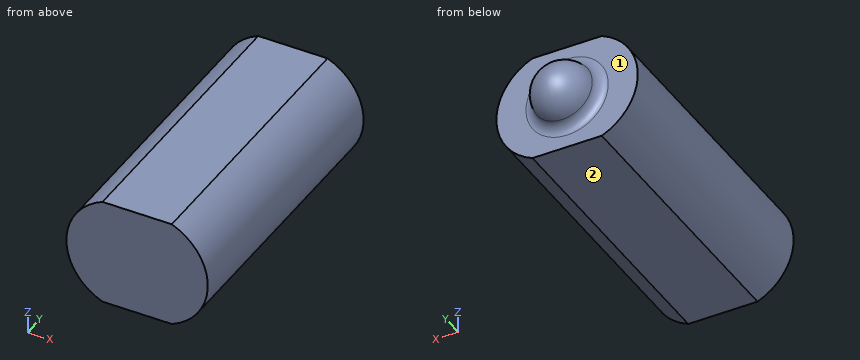
```python
from build123d import *

# Parameters (mm, degrees)
BOSS_EXTRUDE1_DEPTH = 80


with BuildPart() as part:
    # Sketch1 → Boss-Extrude1 (new body)
    with BuildSketch(Plane(origin=(0, 0, 0), x_dir=(1, 0, 0), z_dir=(0, 1, 0))):
        with BuildLine():
            Line((-9.791248996, 15.25), (9.791248996, 15.25))
            ThreePointArc((9.791248996, 15.25), (20, 0), (9.791248996, -15.25))
            Line((9.791248996, -15.25), (-9.791248996, -15.25))
            ThreePointArc((-9.791248996, -15.25), (-20, 0), (-9.791248996, 15.25))
        make_face()
    extrude(amount=BOSS_EXTRUDE1_DEPTH)

    # Sketch4 → Revolve1 (revolve)
    with BuildSketch(Plane(origin=(0, 0, 0), x_dir=(0, 0, -1), z_dir=(1, 0, 0))):
        with BuildLine():
            Line((0, 80), (11.641855063, 80))
            ThreePointArc((11.641855063, 80), (9.61766545, 80.745389743), (8.560304848, 82.625532826))
            ThreePointArc((8.560304848, 82.625532826), (5.623040011, 87.848422876), (0, 89.919057131))
            Line((0, 89.919057131), (0, 80))
        make_face()
    revolve(axis=Axis((0, 80, 0), (0, 1, 0)))


solid = part.part
```
The listing builds one solid part. Answer for the finished solid, in the listing's coordinates (mm). Face numbers are marked on the shaded views. A direction names the side the tool comes from. Give positions to 0.01 mm unless a question says otherwise; leave off trailing zeros. Order: outer loops, then holes, each group sorted by start corner. A loop starts at its lowest first (then second) coordinate and runs counter-clockwise, first axis right, second up.
1) For the marked faces 1 and 2, determine the directions among +Z, -Z, +X, -X, +Y, -Y from which every point of the face is accessible in a straight line to the end or side of a thin tool.
Reported:
face 1: +Y
face 2: -Z, +X, -X, +Y, -Y
2) Find section A-A on y = 23.5. Write down the section's boundary in (x, z), then the cut area to 3 significant figures.
Reported:
outline: (-9.79, -15.25) - (9.79, -15.25) arc R16.49 ccw to (9.79, 15.25) - (-9.79, 15.25) arc R16.49 ccw to start
area: 1,050 mm2
3) Find section B-B on x = 12.5. Write down the section's boundary in (y, z), then the cut area to 3 significant figures.
Reported:
outline: (0, -13.83) - (80, -13.83) - (80, 13.83) - (0, 13.83) - close
area: 2,210 mm2
4) Consider line 1 along Y through (x, z) = (12, 9.5); line 2 along X through (y, z) = (11, -8); line 3 along X through (y, z) = (77, 9.5). Determine where each line is inside the solid, lowest interval first.
Reported:
line 1: y = 0 to 80
line 2: x = -17.93 to 17.93
line 3: x = -16.99 to 16.99
5) Given P1, Ø2, axis at x = 10, z = 5.5, coming from the +Y side; P2, Ø1, axis at y = 51, z = 1.5, coming from the -X side; P3, Ø4, axis at x = -12, y = 44.5, coming from the -Z side, each flat-ended and moving along its own axis, determine where each tip first touches the part or whether it passes through.
Reported:
P1: stops at y = 80.25
P2: stops at x = -19.97
P3: stops at z = -15.16
